Here's how the part is built. I have some questions about the finished solid (model axes, mm). A direction names the side the tool comes from. Coordinates: 2 decimals unless noted, no trailing zeros. Write each loop counter-clockwise with the first axis right and the second up, starting at its lowest first coordinate (ties: lowest second). Pieces come first, ordered by that corner, then holes.
```python
from build123d import *

# Parameters (mm, degrees)
SKETCH_1_W               = 30
SKETCH_1_H               = 7
EXTRUDE_1_DEPTH          = 20
SKETCH_2_W               = 30
SKETCH_2_H               = 15.5
CUT_EXTRUDE_1_DEPTH      = 5
CUT_EXTRUDE_2_DEPTH      = 37.728735344
CUT_EXTRUDE_2_DEPTH_BACK = 37.728735344
SKETCH_4_R               = 1.1
SKETCH_5_W               = 30
SKETCH_5_H               = 2
EXTRUDE_2_DEPTH          = 20
SKETCH_6_W               = 11
SKETCH_6_H               = 2
CUT_EXTRUDE_3_DEPTH      = 2
EXTRUDE_3_DEPTH          = 2
SKETCH_8_R               = 8
EXTRUDE_4_DEPTH          = 3
CUT_EXTRUDE_4_REACH      = 62.033
SKETCH_10_R              = 0.9
FILLET_1_R               = 2


with BuildPart() as part:
    # 草图1 → 凸台-拉伸1 (new body)
    with BuildSketch(Plane(origin=(0, 0, 0), x_dir=(1, 0, 0), z_dir=(0, 1, 0))):
        with Locations((15, -3.5)):
            Rectangle(SKETCH_1_W, SKETCH_1_H)
    extrude(amount=EXTRUDE_1_DEPTH)

    # 草图2 → 切除-拉伸1 (cut)
    with BuildSketch(Plane.XY.offset(7)):
        with Locations((15, 10)):
            Rectangle(SKETCH_2_W, SKETCH_2_H)
    extrude(amount=-CUT_EXTRUDE_1_DEPTH, mode=Mode.SUBTRACT)

    # 草图4 → 切除-拉伸2 (cut, two sides: drawn at the far end of the back side and taken through both)
    with BuildSketch(Plane(origin=(0, 20, 0), x_dir=(1, 0, 0), z_dir=(0, 1, 0)).offset(-CUT_EXTRUDE_2_DEPTH_BACK)):
        with Locations(Location((15, -5.5, 0), (0, 0, 270))):
            Circle(SKETCH_4_R)
    extrude(amount=CUT_EXTRUDE_2_DEPTH + CUT_EXTRUDE_2_DEPTH_BACK, mode=Mode.SUBTRACT)

    # 草图5 → 凸台-拉伸2 (add)
    with BuildSketch(Plane(origin=(0, 0, 0), x_dir=(-1, 0, 0), z_dir=(0, 0, -1))):
        with Locations((-15, 19)):
            Rectangle(SKETCH_5_W, SKETCH_5_H)
    extrude(amount=EXTRUDE_2_DEPTH)

    # 草图6 → 切除-拉伸3 (cut)
    with BuildSketch(Plane(origin=(0, 20, 0), x_dir=(1, 0, 0), z_dir=(0, 1, 0))):
        with Locations((15, 16)):
            Rectangle(SKETCH_6_W, SKETCH_6_H)
        with Locations((15, 4)):
            Rectangle(SKETCH_6_W, SKETCH_6_H)
    extrude(amount=-CUT_EXTRUDE_3_DEPTH, mode=Mode.SUBTRACT)

    # 草图7 → 凸台-拉伸3 (add)
    with BuildSketch(Plane.XZ.offset(-18)):
        with BuildLine():
            Line((0, -12.343145751), (0, -10))
            Line((0, -10), (0, -4.343145751))
            Line((0, -4.343145751), (-23.343145751, -4.343145751))
            Line((-23.343145751, -4.343145751), (-38.907528162, 11.221236661))
            Line((-38.907528162, 11.221236661), (-44.564382411, 5.564382411))
            Line((-44.564382411, 5.564382411), (-29, -10))
            ThreePointArc((-29, -10), (-26.404613209, -11.734182011), (-23.343145751, -12.343145751))
            Line((-23.343145751, -12.343145751), (0, -12.343145751))
        make_face()
    extrude(amount=-EXTRUDE_3_DEPTH)

    # 草图8 → 凸台-拉伸4 (add)
    with BuildSketch(Plane.XZ.offset(-18)):
        with Locations(Location((-44.564382411, 5.564382411, 0), (0, 0, 270))):
            Circle(SKETCH_8_R)
    extrude(amount=-EXTRUDE_4_DEPTH)

    # 草图10 → 切除-拉伸4 (cut, up to next)
    with BuildSketch(Plane(origin=(0, 21, 0), x_dir=(1, 0, 0), z_dir=(0, 1, 0)), mode=Mode.PRIVATE) as cut_extrude_4_sk1:
        with Locations(Location((-38.564382411, -5.564382411, 0), (0, 0, 270))):
            Circle(SKETCH_10_R)
    cut_extrude_4_tool1 = extrude(cut_extrude_4_sk1.sketch, amount=-CUT_EXTRUDE_4_REACH, mode=Mode.PRIVATE) & part.part
    # 草图10 → 切除-拉伸4 (cut, up to next)
    with BuildSketch(Plane(origin=(0, 21, 0), x_dir=(1, 0, 0), z_dir=(0, 1, 0)), mode=Mode.PRIVATE) as cut_extrude_4_sk2:
        with Locations(Location((-44.564382411, -11.564382411, 0), (0, 0, 270))):
            Circle(SKETCH_10_R)
    cut_extrude_4_tool2 = extrude(cut_extrude_4_sk2.sketch, amount=-CUT_EXTRUDE_4_REACH, mode=Mode.PRIVATE) & part.part
    # 草图10 → 切除-拉伸4 (cut, up to next)
    with BuildSketch(Plane(origin=(0, 21, 0), x_dir=(1, 0, 0), z_dir=(0, 1, 0)), mode=Mode.PRIVATE) as cut_extrude_4_sk3:
        with Locations(Location((-50.564382411, -5.564382411, 0), (0, 0, 270))):
            Circle(SKETCH_10_R)
    cut_extrude_4_tool3 = extrude(cut_extrude_4_sk3.sketch, amount=-CUT_EXTRUDE_4_REACH, mode=Mode.PRIVATE) & part.part
    # 草图10 → 切除-拉伸4 (cut, up to next)
    with BuildSketch(Plane(origin=(0, 21, 0), x_dir=(1, 0, 0), z_dir=(0, 1, 0)), mode=Mode.PRIVATE) as cut_extrude_4_sk4:
        with Locations(Location((-44.564382411, 0.435617589, 0), (0, 0, 270))):
            Circle(SKETCH_10_R)
    cut_extrude_4_tool4 = extrude(cut_extrude_4_sk4.sketch, amount=-CUT_EXTRUDE_4_REACH, mode=Mode.PRIVATE) & part.part
    add(cut_extrude_4_tool1.solids().sort_by_distance((-38.564382, 21, 5.564382))[0], mode=Mode.SUBTRACT)
    add(cut_extrude_4_tool2.solids().sort_by_distance((-44.564382, 21, 11.564382))[0], mode=Mode.SUBTRACT)
    add(cut_extrude_4_tool3.solids().sort_by_distance((-50.564382, 21, 5.564382))[0], mode=Mode.SUBTRACT)
    add(cut_extrude_4_tool4.solids().sort_by_distance((-44.564382, 21, -0.435618))[0], mode=Mode.SUBTRACT)

    # 圆角1
    fillet_1_edges = [part.edges().sort_by_distance(p)[0] for p in [
        (30, 1.125, 7),
        (0, 1.125, 7),
        (30, 19, -20),
        (0, 19, -20),
        (30, 18.875, 7),
        (0, 18.875, 7),
    ]]
    fillet(fillet_1_edges, radius=FILLET_1_R)


solid = part.part
```
1) Imagine slicing it at B-B on z = 3. Please give me the cut outline in (x, y), then the cut area to 3 significant figures.
Values follow:
outline: (-52.14, 18) - (-30.69, 18) - (-30.69, 20) - (-36.99, 20) - (-36.99, 21) - (-52.14, 21) - close; (0, 0) - (30, 0) - (30, 2.25) - (0, 2.25) - close; (0, 17.75) - (30, 17.75) - (30, 20) - (0, 20) - close
area: 193 mm2
2) Will these pins go through, and if not, where does the flat tip stop? pin 1 (6 mm diameter, centred on x = -31.5, z = -3, fed in from -Y); pin 2 (2 mm diameter, centred on y = 19, z = -14, fed in from -X); pin 3 (2.5 mm diameter, centred on x = 14.5, y = 1.5, fed in from +Z); pin 4 (8 mm diameter, centred on x = -5, y = 13.5, fed in from -Z).
Values follow:
pin 1: stops at y = 18
pin 2: stops at x = 0
pin 3: stops at z = 7
pin 4: passes through
3) We'd pull the mould along Z, two halves only. Please class faces 1 (the face through (9.5, 19, -16)), 2 (the face through (15, 10, 2)), 3 (the face through (29.4, 19.01, -19.43)): pulls with the +Z half, pulls with the -Z half, needs draft (parallel to the pull), parting line crosses it, or undercut.
Values follow:
face 1: undercut
face 2: pulls with the +Z half
face 3: pulls with the -Z half
4) I need wall thicknesses on probe 1 along Z at (x, y) = (15, 18.8); probe 2 along Y at (x, z) = (2, 6); probe 3 along Z at (x, y) = (10, 2). Which ranges of each line are inside material? Lowest first, please.
Values follow:
probe 1: z = -20 to -17, -15 to -5, -3 to 4.4, 6.6 to 7
probe 2: y = 0 to 2.25, 17.75 to 20
probe 3: z = 0 to 7
5) On a 3-axis mill with a long thin cutter (end or side, diameter ignored), from which of +Z, -Z, +X, -X, +Y, -Y can I reach the whole of each face in a straight line? I mean faces 4 (the face through (15, 2.25, 4)), 5 (the face through (-12, 19, -12.343)), 6 (the face through (9.5, 19, -4)). Say none if no direction works.
Values follow:
face 4: +Z, +X, -X
face 5: -Z, -X, +Y, -Y
face 6: +Y, -Y
6) Imagine slicing it at D-D on x = -9.5. Please give me the cut outline in (y, z), then the cut area to 3 significant figures.
Values follow:
outline: (18, -12.34) - (20, -12.34) - (20, -4.34) - (18, -4.34) - close
area: 16.0 mm2
7) Imagine slicing it at C-C on y = 5. Please give me the cut outline in (x, z).
Values follow:
outline: (0, 0) - (30, 0) - (30, 2) - (0, 2) - close
8) Imagine slicing it at A-A on x = 13. Please give me the cut outline in (y, z), then the cut area to 3 significant figures.
Values follow:
outline: (0, 0) - (18, 0) - (18, -3) - (20, -3) - (20, 7) - (17.75, 7) - (17.75, 2) - (2.25, 2) - (2.25, 7) - (0, 7) - close; (18, -20) - (20, -20) - (20, -17) - (18, -17) - close; (18, -15) - (20, -15) - (20, -5) - (18, -5) - close
area: 94.5 mm2
